Geometry check sheet. Reference: the model listing, model coordinates, mm. Coordinates: 2 decimals unless noted, no trailing zeros. Loops run counter-clockwise (first coordinate to the right, second up) from the corner with the lowest first, then second, coordinate; pieces in that order, holes last.
from build123d import *

# Parameters (mm, degrees)
SKETCH1_R           = 1.25
SKETCH1_R_2         = 2
BOSS_EXTRUDE1_DEPTH = 4.5
FILLET5_R           = 2.5


with BuildPart() as part:
    # Sketch1 → Boss-Extrude1 (new body)
    with BuildSketch(Plane(origin=(0, 0, 0), x_dir=(1, 0, 0), z_dir=(0, 1, 0))):
        with BuildLine():
            Line((-6, 50), (0, 50))
            Line((0, 50), (0, 5))
            ThreePointArc((0, 5), (-3.535533906, -3.535533906), (5, 0))
            Line((5, 0), (5, 50))
            Line((5, 50), (44.2, 50))
            Line((44.2, 50), (44.2, 0))
            ThreePointArc((44.2, 0), (52.735533906, -3.535533906), (49.2, 5))
            Line((49.2, 5), (49.2, 50))
            Line((49.2, 50), (49.2, 60))
            Line((49.2, 60), (49.2, 104))
            ThreePointArc((49.2, 104), (52.735533906, 112.535533906), (44.2, 109))
            Line((44.2, 109), (44.2, 60))
            Line((44.2, 60), (-1, 60))
            Line((-1, 60), (-1, 115.2))
            ThreePointArc((-1, 115.2), (-9.535533906, 118.735533906), (-6, 110.2))
            Line((-6, 110.2), (-6, 60))
            Line((-6, 60), (-6, 50))
        make_face()
        Circle(SKETCH1_R, mode=Mode.SUBTRACT)
        with Locations((49.2, 0)):
            Circle(SKETCH1_R, mode=Mode.SUBTRACT)
        with Locations((30.2, 55)):
            Circle(SKETCH1_R_2, mode=Mode.SUBTRACT)
        with Locations((37.2, 55)):
            Circle(SKETCH1_R_2, mode=Mode.SUBTRACT)
        with Locations((44.2, 55)):
            Circle(SKETCH1_R_2, mode=Mode.SUBTRACT)
        with Locations((-6, 115.2)):
            Circle(SKETCH1_R, mode=Mode.SUBTRACT)
        with Locations((49.2, 109)):
            Circle(SKETCH1_R, mode=Mode.SUBTRACT)
    extrude(amount=BOSS_EXTRUDE1_DEPTH)

    # Fillet5
    fillet5_edges = [part.edges().sort_by_distance(p)[0] for p in [
        (-1, 2.25, -60),
        (44.2, 2.25, -60),
        (49.2, 2.25, -104),
        (49.2, 2.25, -5),
        (44.2, 2.25, -50),
        (5, 2.25, -50),
        (0, 2.25, -5),
        (0, 2.25, -50),
        (-6, 2.25, -50),
        (-6, 2.25, -110.2),
    ]]
    fillet(fillet5_edges, radius=FILLET5_R)


solid = part.part
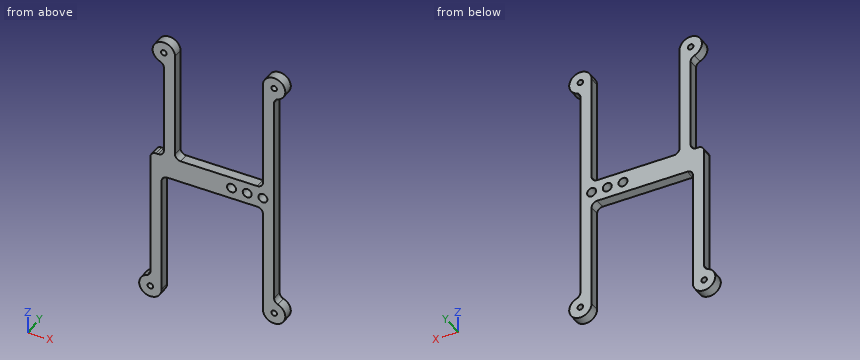
1) Section check C-C on y = 3.05. Count the separate pieces of the cut face and the enclosed holes in it, and give its area (3 significant figures).
Data:
separate pieces: 1
enclosed holes: 7
area: 1,760 mm2
2) Section check A-A on x = 30.2. Record the cut outline in (y, z), and give its area (3 significant figures).
Data:
outline: (0, -60) - (4.5, -60) - (4.5, -57) - (0, -57) - close; (0, -53) - (4.5, -53) - (4.5, -50) - (0, -50) - close
area: 27.0 mm2
3) Material ranges on probe 1 along X at (y, z) = (2.15, -55); probe 2 along X at (y, z) = (2.5, -115.2); probe 3 along Z at (x, y) = (30.2, 3.25), recorded low to high.
Data:
probe 1: x = -6 to 28.2, 32.2 to 35.2, 39.2 to 42.2, 46.2 to 49.2
probe 2: x = -11 to -7.25, -4.75 to -1
probe 3: z = -60 to -57, -53 to -50
4) Section check B-B on z = -9. Record the cut outline in (x, y).
Data:
outline: (0, 0) - (5, 0) - (5, 4.5) - (0, 4.5) - close; (44.2, 0) - (49.2, 0) - (49.2, 4.5) - (44.2, 4.5) - close
5) Section check D-D on z = -55. Record the cut outline in (x, y).
Data:
outline: (-6, 0) - (28.2, 0) - (28.2, 4.5) - (-6, 4.5) - close; (32.2, 0) - (35.2, 0) - (35.2, 4.5) - (32.2, 4.5) - close; (39.2, 0) - (42.2, 0) - (42.2, 4.5) - (39.2, 4.5) - close; (46.2, 0) - (49.2, 0) - (49.2, 4.5) - (46.2, 4.5) - close
6) Depth check by flat-ended pin: pin 1 (1.3 mm diameter, centred on y = 3, z = -19, fed in from +X); pin 2 (1.3 mm diameter, centred on y = 1, z = -78.5, fed in from -X); pin 3 (2 mm diameter, centred on y = 2, z = -17.5, fed in from -X). Enter the tip coordinate at first touch or a pass-through.
Data:
pin 1: stops at x = 49.2
pin 2: stops at x = -6
pin 3: stops at x = 0
